Verification items for the finished model (mm, model axes). A direction names the side the tool comes from. Give positions to 0.01 mm unless a question says otherwise; leave off trailing zeros. Order: outer loops, then holes, each group sorted by start corner. A loop starts at its lowest first (then second) coordinate and runs counter-clockwise, first axis right, second up. Notation, with made-up numbers: (31.25, -16) - (40.25, -16) arc R29 cw to (40.25, 11) - close; hole circle Ø11 at (3.5, 47). An arc over 180 degrees is marked (long way). Answer as a JSON object with one key per item and string values. Group by question number.
(1) Thickness scan on line 1 (Y direction, x = 60.5, z = -1.8); line 2 (Y direction, x = -25, z = -0.95); line 3 (Y direction, x = 46, z = -0.35). Record the ranges inside material, lowest first.
(2) Access from +Z, -Z, +X, -X, +Y, -Y to the whole of each face (thin tool, end or side, straight path). Record for faces 4 (the face through (61, 26.25, -1)), 5 (the face through (-1, 0, -2)).
(3) Section check D-D (y = -24). Record the boundary of the cut face in (x, z) (3 decimals).
(4) Section check B-B (y = 0). Record the boundary of the cut face in (x, z), then the cut area to 3 significant figures.
(5) Section check C-C (z = -0.15). Record the boundary of the cut face in (x, y) (3 decimals), then the cut area to 3 significant figures.
(6) Section check A-A (x = 46). Record the boundary of the cut face in (y, z), then the cut area to 3 significant figures.
(7) Mould release check, pull along Y, two halves, no side actions. Record for faces 1 (the face through (59.535, 22, -1)), 2 (the face through (-1, -30, 0)), 3 (the face through (-65, 0, 0)): +Y half, -Y half, draft (parallel to the pull), parting line (faces both ways), or undercut.
```python
from build123d import *

# Parameters (mm, degrees)
SKETCH1_W           = 130
SKETCH1_H           = 60
SKETCH1_R           = 5
SKETCH1_R_2         = 2.83
SKETCH1_W_2         = 3.53
SKETCH1_H_2         = 9.2
BOSS_EXTRUDE1_DEPTH = 2
CHAMFER1_SIZE       = 0.5
CHAMFER1_SIZE2      = 1.5


with BuildPart() as part:
    # Sketch1 → Boss-Extrude1 (new, symmetric)
    with BuildSketch(Plane.XY):
        Rectangle(SKETCH1_W, SKETCH1_H)
        with Locations((-25, 0)):
            Circle(SKETCH1_R, mode=Mode.SUBTRACT)
        with Locations((46, -24)):
            Circle(SKETCH1_R_2, mode=Mode.SUBTRACT)
        with Locations((61.3, 21.65)):
            Rectangle(SKETCH1_W_2, SKETCH1_H_2, mode=Mode.SUBTRACT)
        with Locations((61.3, -21.65)):
            Rectangle(SKETCH1_W_2, SKETCH1_H_2, mode=Mode.SUBTRACT)
    extrude(amount=BOSS_EXTRUDE1_DEPTH, both=True)

    # Chamfer1
    chamfer1_edges = [part.edges().sort_by_distance(p)[0] for p in [
        (59.535, -21.65, 2),
        (61.3, -26.25, 2),
        (63.065, -21.65, 2),
        (61.3, -17.05, 2),
        (43.17, -24, 2),
        (-30, 0, 2),
        (59.535, 21.65, 2),
        (61.3, 17.05, 2),
        (63.065, 21.65, 2),
        (61.3, 26.25, 2),
    ]]
    chamfer1_side = [part.faces().sort_by_distance(p)[0] for p in [
        (-0.416106653, 0.079128468, 2),
    ]]
    chamfer(chamfer1_edges, length=CHAMFER1_SIZE, length2=CHAMFER1_SIZE2, reference=chamfer1_side[0])


solid = part.part
```
Solutions:
{
 "1": {"line 1": "y = -30 to -26.25, -17.05 to 17.05, 26.25 to 30", "line 2": "y = -30 to -5, 5 to 30", "line 3": "y = -30 to -26.83, -21.17 to 30"},
 "2": {"face 4": "+Z, -Z", "face 5": "-Z, +X, -X, +Y, -Y"},
 "3": {"outline": "(-65, -2) - (43.17, -2) - (43.17, 0.5) - (42.67, 2) - (-65, 2) - close; (48.83, -2) - (59.535, -2) - (59.535, 0.5) - (59.035, 2) - (49.33, 2) - (48.83, 0.5) - close; (63.065, -2) - (65, -2) - (65, 2) - (63.565, 2) - (63.065, 0.5) - close"},
 "4": {"outline": "(-65, -2) - (-30, -2) - (-30, 0.5) - (-30.5, 2) - (-65, 2) - close; (-20, -2) - (65, -2) - (65, 2) - (-19.5, 2) - (-20, 0.5) - close", "area": "479 mm2"},
 "5": {"outline": "(-65, -30) - (65, -30) - (65, 30) - (-65, 30) - close; hole circle Ø10 at (-25, 0); hole circle Ø5.66 at (46, -24); hole (59.535, -26.25) - (63.065, -26.25) - (63.065, -17.05) - (59.535, -17.05) - close; hole (59.535, 17.05) - (63.065, 17.05) - (63.065, 26.25) - (59.535, 26.25) - close", "area": "7,630 mm2"},
 "6": {"outline": "(-30, -2) - (-26.83, -2) - (-26.83, 0.5) - (-27.33, 2) - (-30, 2) - close; (-21.17, -2) - (30, -2) - (30, 2) - (-20.67, 2) - (-21.17, 0.5) - close", "area": "217 mm2"},
 "7": {"face 1": "undercut", "face 2": "-Y half", "face 3": "draft"}
}
